```python
from build123d import *

# Parameters (mm, degrees)
BOSS_EXTRU_1_DEPTH      = 5
CONG_2_R                = 25
ESQUISSE5_W             = 40
ESQUISSE5_H             = 15
ENL_V_MAT_EXTRU_1_DEPTH = 5
CONG_3_R                = 10
ESQUISSE2_R             = 1
ENL_V_MAT_EXTRU_5_DEPTH = 10
D_GAGEMENT_M21_D        = 2.4
ESQUISSE9_W             = 25
ESQUISSE9_H             = 10
ENL_V_MAT_EXTRU_6_DEPTH = 5


with BuildPart() as part:
    # Esquisse1 → Boss.-Extru.1 (new body)
    with BuildSketch(Plane.XY):
        Polygon((0, 0), (0, 54), (-8, 54), (-8, 80), (0, 80), (0, 140), (120, 140), (120, 130), (30, 130), (30, 80), (70, 80), (70, 0), (62, 0), (62, 54), (8, 54), (8, 0), align=None)
    extrude(amount=BOSS_EXTRU_1_DEPTH)

    # Congé2
    cong_2_edges = [part.edges().sort_by_distance(p)[0] for p in [
        (30, 130, 2.5),
    ]]
    fillet(cong_2_edges, radius=CONG_2_R)

    # Esquisse5 → Enlèv. mat.-Extru.1 (cut)
    with BuildSketch(Plane.XY.offset(5)):
        with Locations((50, 72.5)):
            Rectangle(ESQUISSE5_W, ESQUISSE5_H)
    extrude(amount=-ENL_V_MAT_EXTRU_1_DEPTH, mode=Mode.SUBTRACT)

    # Congé3
    cong_3_edges = [part.edges().sort_by_distance(p)[0] for p in [
        (70, 65, 2.5),
        (30, 65, 2.5),
    ]]
    fillet(cong_3_edges, radius=CONG_3_R)

    # Esquisse2 → Enlèv. mat.-Extru.5 (cut)
    with BuildSketch(Plane.XY.offset(5)):
        with Locations((4, 4)):
            Circle(ESQUISSE2_R)
        with Locations((66, 4)):
            Circle(ESQUISSE2_R)
    extrude(amount=-ENL_V_MAT_EXTRU_5_DEPTH, mode=Mode.SUBTRACT)

    # Dégagement M21 (through all)
    with Locations(Plane.XY.offset(5)):
        with Locations((4, 4), (66, 4)):
            Hole(D_GAGEMENT_M21_D / 2)

    # Esquisse9 → Enlèv. mat.-Extru.6 (cut)
    with BuildSketch(Plane.XY.offset(5)):
        with Locations((107.5, 135)):
            Rectangle(ESQUISSE9_W, ESQUISSE9_H)
    extrude(amount=-ENL_V_MAT_EXTRU_6_DEPTH, mode=Mode.SUBTRACT)


solid = part.part
```
Read the model definition and answer for the solid it produces. Units are mm, in the model's axes. A direction names the side the tool comes from. Coordinates: 2 decimals unless noted, no trailing zeros. Write each loop counter-clockwise with the first axis right and the second up, starting at its lowest first coordinate (ties: lowest second). Pieces come first, ordered by that corner, then holes. Notation, with made-up numbers: (77.25, 26.5) -> (114.25, 26.5) arc R13 ccw to (114.25, 47.5) -> close; hole circle Ø4 at (-40, 27). An arc over 180 degrees is marked (long way). Write item = value, one per line.
(1) Straight lines are drawn through the part: L1, parallel to Y at x = 66, z = 2.55; L2, parallel to X at y = 9, z = 4.3; L3, parallel to Y at x = 54, z = 1.2. For each, find the intervals that lie inside material, in ascending order. Write a range as from..to.
From the geometry:
L1 = 0..2.8, 5.2..63, 130..140
L2 = 0..8, 62..70
L3 = 54..65, 129.98..140
(2) Section C-C on y = 97.5 is taken. Write down the section's boundary in (x, z), plus the area to 3 significant figures.
From the geometry:
outline = (0, 0) -> (30, 0) -> (30, 5) -> (0, 5) -> close
area = 150 mm2
(3) Given pin 1 Ø2 at (x, z) = (54, 3.5) entering from -Y; pin 2 Ø1.5 at (y, z) = (27, 2) entering from -X; pin 3 Ø1.5 at (y, z) = (91, 2) entering from +X; pin 4 Ø3 at (x, y) = (66, 4) entering from -Z, each flat-ended and moving along its own axis, determine where each tip first touches the part or whether it passes through.
From the geometry:
pin_1 = 54
pin_2 = 0
pin_3 = 30
pin_4 = 0
(4) Which of the six approach directions +Z, -Z, +X, -X, +Y, -Y give full straight-line access (tool end or side, diameter ignored) to faces 4 (the face through (70, 28, 2)), 5 (the face through (33.01, 67.85, 2.46)), 6 (the face through (8, 27, 2)), 7 (the face through (-4, 80, 2)), 8 (the face through (0, 27, 2))?
From the geometry:
face_4 = +Z, -Z, +X, -Y
face_5 = +Z, -Z, +X
face_6 = +Z, -Z, -Y
face_7 = +Z, -Z, -X, +Y
face_8 = +Z, -Z, -X, -Y
(5) For a pull along X with two mould halves and no side action, classify faces 1 (the face through (62, 27, 2)), 2 (the face through (95, 135, 3)), 3 (the face through (0, 110, 2)) as +X half, -X half, draft (parallel to the pull), parting line (faces both ways), or undercut.
From the geometry:
face_1 = undercut
face_2 = +X half
face_3 = -X half
(6) Section B-B on x = 85.5 is taken. Write down the section's boundary in (y, z).
From the geometry:
outline = (130, 0) -> (140, 0) -> (140, 5) -> (130, 5) -> close
(7) Section A-A on z = 2.3 is taken. Write down the section's boundary in (x, y).
From the geometry:
outline = (-8, 54) -> (0, 54) -> (0, 0) -> (8, 0) -> (8, 54) -> (62, 54) -> (62, 0) -> (70, 0) -> (70, 55) arc R10 ccw to (60, 65) -> (40, 65) arc R10 cw to (30, 75) -> (30, 105) arc R25 cw to (55, 130) -> (95, 130) -> (95, 140) -> (0, 140) -> (0, 80) -> (-8, 80) -> close; hole circle Ø2.4 at (4, 4); hole circle Ø2.4 at (66, 4)
